Source: CAD feature listing. Evaluate the final solid. Frame: model axes, mm. Face numbers are marked on the shaded views. A direction names the side the tool comes from. Round coordinates to 2 decimals unless told otherwise and drop trailing zeros. Order: outer loops, then holes, each group sorted by start corner. A loop starts at its lowest first (then second) coordinate and runs counter-clockwise, first axis right, second up. Notation, with made-up numbers: (51, 19.5) - (94, 19.5) arc R6 ccw to (94, 30.5) - close; hole circle Ø6 at (50.25, 36). An arc over 180 degrees is marked (long way). Return JSON: item names as keys, results as strings. Group by question number.
1) Section B-B, the plane z = 328.5. Return loops of the section in (x, y), plus the area to 3 significant figures.
2) Access query for the marked faces 1 and 2. Directions: +Z, -Z, +X, -X, +Y, -Y. A direction counts if a zero-diameter tool reaches every point of the face in a straight line with its end or side. Return the directions, or none.
3) Mould query, pull axis Z, two halves, no side actions, for the marked faces 3, 4, 5 and 6. Classes: pulls with the +Z half, pulls with the -Z half, needs draft (parallel to the pull), parting line crosses it, or undercut.
4) Section C-C, the plane x = -23.5. Return loops of the section in (y, z).
5) Contact query for flat-ended pins moving along their axis: P1, Ø5, axis at x = -21, z = 398, coming from the -Y side; P2, Ø4, axis at y = 190, z = 1041, coming from the -X side; P3, Ø5, axis at x = -37.5, z = 1005.5, coming from the +Y side. Output: stop coordinate, or through.
6) Section D-D, the plane y = 208. Return loops of the section in (x, z), plus the area to 3 significant figures.
7) Section A-A, the plane y = 307. Return loops of the section in (x, z), plus the area to 3 significant figures.
8) Ray query, line 1 (Z direction, x = -70, y = 222.5); line 2 (Y direction, x = -19.5, z = 748); line 3 (X direction, y = 172, z = 145). Return the intervals inside material, ascending. Write a range as from..to.
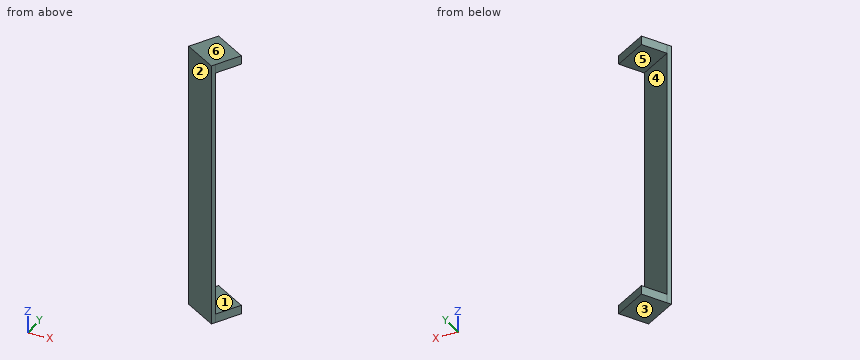
```python
from build123d import *

# Parameters (mm, degrees)
BOSS_EXTRUDE1_DEPTH = 1220
SKETCH4_W           = 169.510039034
SKETCH4_H           = 40
BOSS_EXTRUDE3_DEPTH = 120


with BuildPart() as part:
    # Sketch1 → Boss-Extrude1 (new body)
    with BuildSketch(Plane.XY):
        Polygon((0, 146.8), (10, 164.120508076), (-136.8, 248.875527593), (-146.8, 231.555019517), align=None)
    extrude(amount=BOSS_EXTRUDE1_DEPTH)

    # Sketch4 → Boss-Extrude3 (add)
    with BuildSketch(Plane(origin=(73.566264638, 127.420508076, 0), x_dir=(0.86602540378444, -0.4999999999999976, 0), z_dir=(0.4999999999999976, 0.86602540378444, 0))):
        with Locations((-158.155019517, -1200)):
            Rectangle(SKETCH4_W, SKETCH4_H)
        with Locations((-158.155019517, -20)):
            Rectangle(SKETCH4_W, SKETCH4_H)
    extrude(amount=BOSS_EXTRUDE3_DEPTH)


solid = part.part
```
Geometry check:
{
 "1": {"outline": "(-146.8, 231.56) - (0, 146.8) - (10, 164.12) - (-136.8, 248.88) - close", "area": "3,390 mm2"},
 "2": {"face 1": "+X, +Y", "face 2": "+Z, -Z, -X, -Y"},
 "3": {"face 3": "pulls with the -Z half", "face 4": "undercut", "face 5": "undercut", "face 6": "pulls with the +Z half"},
 "4": {"outline": "(160.37, 0) - (322.03, 0) - (322.03, 40) - (183.46, 40) - (183.46, 1180) - (322.03, 1180) - (322.03, 1220) - (160.37, 1220) - close"},
 "5": {"P1": "y = 157.48", "P2": "x = -78.29", "P3": "y = 192.99"},
 "6": {"outline": "(-106, 0) - (35.33, 0) - (35.33, 40) - (-66, 40) - (-66, 1180) - (35.33, 1180) - (35.33, 1220) - (-106, 1220) - close", "area": "56,900 mm2"},
 "7": {"outline": "(-103.24, 0) - (2.53, 0) - (2.53, 40) - (-103.24, 40) - close; (-103.24, 1180) - (2.53, 1180) - (2.53, 1220) - (-103.24, 1220) - close", "area": "8,460 mm2"},
 "8": {"line 1": "0..40, 1180..1220", "line 2": "158.06..181.15", "line 3": "-43.65..-3.65"}
}
